Build history of the part. All positions in model axes, mm. A direction names the side the tool comes from. Round coordinates to 2 decimals unless told otherwise and drop trailing zeros. Order: outer loops, then holes, each group sorted by start corner. A loop starts at its lowest first (then second) coordinate and runs counter-clockwise, first axis right, second up. Notation, with made-up numbers: (-19.5, -11) -> (-11.5, -11) arc R29 ccw to (-11.5, 15) -> close; hole circle Ø11 at (-24, -13). An arc over 180 degrees is marked (long way). Write item = value, one per line.
Autodesk Inventor part; units mm, degrees
ref_plane "YZ Plane" through (0, 0, 0) normal (1, 0, 0) x (0, 1, 0)
ref_plane "XZ Plane" through (0, 0, 0) normal (0, 1, 0) x (-1, 0, 0)
ref_plane "XY Plane" through (0, 0, 0) normal (0, 0, 1) x (1, 0, 0)
sketch "Эскиз1" plane through (0, 0, 0) normal (0, 0, 1) x (1, 0, 0)
  line L0 (-26.5, 0) -> (26.5, 0)
  line L1 (-26.5, -14.3929) -> (-26.5, -27.5)
  line L2 (-25.5, -28.5) -> (-24, -28.5)
  line L3 (-26.5, -14.3929) -> (-25.5, -14.125)
  line L4 (-25.5, -14.125) -> (25.5, -14.125)
  line L5 (-25.5, -28.5) -> (-26.5, -27.5)
  line L6 (-21, -31.5) -> (-21, -36.75)
  arc A0 (-21, -31.5) -> (-24, -28.5) centre (-24, -31.5) ccw
  line L7 (-21, -36.75) -> (-0.5, -36.75)
  line L8 (-0.5, -36.75) -> (-0.5, -30.5)
  line L9 (-0.5, -30.5) -> (1, -29)
  line L10 (1, -29) -> (1, -23)
  line L11 (1, -23) -> (5, -23)
  line L12 (5, -23) -> (5, -29)
  line L13 (5, -29) -> (6.5, -30.5)
  line L14 (6.5, -30.5) -> (6.5, -45.125)
  line L15 (6.5, -45.125) -> (26.5, -45.125)
  line L16 (26.5, -45.125) -> (26.5, -14.3929)
  line L17 (26.5, -14.3929) -> (25.5, -14.125)
  point P0 (0, 0)
  point P1 (0, 0)
  point P2 (-26.5, -28.5)
  dimension "d0" = 53
  dimension "d1" = 28.25
  dimension "d2" = 15
  dimension "d3" = 57
  dimension "d4" = 1
  dimension "d5" = 1
  dimension "d6" = 45
  dimension "d7" = 3
  dimension "d8" = 73.5
  dimension "d9" = 5.5
  dimension "d10" = 7
  dimension "d11" = 4
  dimension "d12" = 46
  dimension "d13" = 21.5
  dimension "d14" = 20
  dimension "d15" = 58
  dimension "d16" = 45
  dimension "d17" = 15
  dimension "d18" = 1
  dimension "d19" = 90.25
revolve "Вращение1" add sketch "Эскиз1" angle 360 about axis through (-26.5, 0, 0) along (1, 0, 0)
properties part number "71. Блок шестерен заднего хода"
Q1. Cut at C-C, the plane x = 16. List the corners of the cut face in (y, z) (3 decimals).
Check values:
outline = circle Ø90.25 at (0, 0); hole circle Ø28.25 at (0, 0)
Q2. Cut at A-A, the plane z = -34. List the corners of the cut face in (x, y), and give its area (3 significant figures).
Check values:
outline = (-21, -13.95) -> (-0.5, -13.95) -> (-0.5, 13.95) -> (-21, 13.95) -> close; (6.5, -29.67) -> (26.5, -29.67) -> (26.5, 29.67) -> (6.5, 29.67) -> close
area = 1,760 mm²
Q3. Cut at B-B, the plane x = -14.5. List the corners of the cut face in (y, z) (3 decimals), and give its area (3 significant figures).
Check values:
outline = circle Ø73.5 at (0, 0); hole circle Ø28.25 at (0, 0)
area = 3,620 mm²
Q4. Mould opens along Y. For faces 1 (the face through (26.5, 11, -11)), 2 (the face through (0.357, -7.594, -11.91)), 3 (the face through (3.028, 2.994, -22.804)) say: released by +Y, released by -Y, zero draft, split by the parting line, or undercut.
Check values:
face_1 = zero draft
face_2 = undercut
face_3 = split by the parting line
Q5. Probe probe 1 along Z at (x, y) = (-1.5, 0) (3 decimals); probe 2 along X at (y, z) = (-32.5, -13); probe 3 along X at (y, z) = (40, 1.5). List the from-to ranges inside material, lowest first.
Check values:
probe_1 = -36.75 to -14.125, 14.125 to 36.75
probe_2 = -21 to -0.5, 6.5 to 26.5
probe_3 = 6.5 to 26.5
Q6. Flat gauge pins, fed straight in: pin 1 (5 mm diameter, centred on x = 1, z = 3, fed in from -Y); pin 2 (3 mm diameter, centred on x = 18, y = 20, fed in from +Z); pin 3 (2 mm diameter, centred on x = 16.5, y = 2, fed in from -Z). Where does each tip first touch, or does it go through?
Check values:
pin_1 = -36.74
pin_2 = 41.16
pin_3 = -45.11
Q7. Cut at D-D, the plane z = 39. List the corners of the cut face in (x, y).
Check values:
outline = (6.5, -22.7) -> (26.5, -22.7) -> (26.5, 22.7) -> (6.5, 22.7) -> close
Q8. Which spindle directions (+Z, -Z, +X, -X, +Y, -Y) get a long thin tool onto all of the face, cutting with end or side? Do faces 4 (the face through (-26.5, -12, 12)), 5 (the face through (6.5, -9.4, 29.5)), 6 (the face through (-24.74, -26.327, 10.916)). Say none if no direction does.
Check values:
face_4 = +Z, -Z, -X, +Y, -Y
face_5 = none
face_6 = -X
